Design review of the part built by this model. Coordinates are the model's own, in mm. A direction names the side the tool comes from. Give positions to 0.01 mm unless a question says otherwise; leave off trailing zeros. Loops run counter-clockwise (first coordinate to the right, second up) from the corner with the lowest first, then second, coordinate; pieces in that order, holes last. Notation, with made-up numbers: (65, 78.5) -> (75, 78.5) arc R19 cw to (75, 95.5) -> close; hole circle Ø10 at (78.25, 51.5). An arc over 180 degrees is marked (long way). Use CSV: the item, a comma, the result in double quotes. Start each with the question number.
Item 1: Clearance check with flat-ended pins moving along their axes: pin 1 (0.9 mm diameter, centred on y = -2.5, z = -4, fed in from +X) (3 decimals); pin 2 (6 mm diameter, centred on y = 17, z = -8.5, fed in from +X); pin 3 (1.4 mm diameter, centred on x = -5, y = -3.5, fed in from -Z); pin 4 (1 mm diameter, centred on y = -3.5, z = -5.5, fed in from +X). State where each tip first meets the part, or that it passes through.
Item 2: We need section C-C (y = 5.5). State the section outline as (x, z) points.
Item 3: Wall thickness on line 1 along Y through (x, z) = (2.5, -8.25); line 2 along Z through (x, y) = (10.75, 8); line 3 along Z through (x, y) = (4.5, -6): over which ranges is each line inside the solid? List them lowest first. Write a range as from..to.
Item 4: We need section A-A (y = -1). State the section outline as (x, z) points (3 decimals).
Item 5: We need section B-B (x = 0). State the section outline as (y, z) points.
Item 6: The part is to be moulded in two halves that separate along X. For faces 6 (the face through (-1.5, 15.1, 11.4)), 7 (the face through (6.875, -4, -4)), 8 (the face through (-5, -4, 3.6)), 9 (the face through (2.125, -4, -4)), say which applies: +X half, -X half, draft (parallel to the pull), parting line (faces both ways), or undercut.
Item 7: For faces 1 (the face through (11, 7, -1.1)), 2 (the face through (-9, 14.5, -5)), 3 (the face through (-5, -4, -4.4)), 4 (the face through (-6.875, -4, -4)), 5 (the face through (-4, -4, -3.6)), list the 3-axis set-ups (+Z, -Z, +X, -X, +Y, -Y) from which the entire face can be reached by the end or side of a thin tool; tool diameter is ignored.
Autodesk Inventor part; units mm, degrees
ref_plane "YZ Plane" through (0, 0, 0) normal (1, 0, 0) x (0, 1, 0)
ref_plane "XZ Plane" through (0, 0, 0) normal (0, 1, 0) x (-1, 0, 0)
ref_plane "XY Plane" through (0, 0, 0) normal (0, 0, 1) x (1, 0, 0)
sketch "Sketch1" plane through (0, 0, 0) normal (0, 1, 0) x (-1, 0, 0)
  circle A0 centre (0, 0) radius 9.9
  line L0 (-9.8387, 1.1) -> (-12.0387, 1.1)
  line L1 (-12.0387, 1.1) -> (-12.0387, -1.1)
  line L2 (-12.0387, -1.1) -> (-9.8387, -1.1)
  point P0 (-12.0387, 0)
  dimension "d0" = 19.8
  dimension "d1" = 2.2
  dimension "d2" = 2.2
extrude "Extrusion1" add sketch "Sketch1" along normal blind 14.5
sketch "Sketch2" plane through (0, 14.5, 0) normal (0, 1, 0) x (1, 0, 0)
  circle A0 centre (0, 0) radius 11.5
  dimension "d5" = 23
extrude "Extrusion2" add sketch "Sketch2" along normal blind 2
chamfer "Chamfer1" distance 0.8 angle 45 1 edges at (-11.5, 16.5, 0)
sketch "Sketch3" plane through (0, 16.5, 0) normal (0, 1, 0) x (1, 0, 0)
  circle A0 centre (0, 0) radius 10.2
  dimension "d11" = 20.4
extrude "Extrusion3" add sketch "Sketch3" along normal blind 7.5
sketch "Sketch4" plane through (0, 0, 0) normal (0, -1, 0) x (1, 0, 0)
  line L0 (-6.875, -4.4) -> (-2.125, -4.4)
  line L1 (-2.125, -4.4) -> (-2.125, -3.6)
  line L2 (-2.125, -3.6) -> (-6.875, -3.6)
  line L3 (-6.875, -3.6) -> (-6.875, -4.4)
  line L4 (2.125, -4.4) -> (6.875, -4.4)
  line L5 (6.875, -4.4) -> (6.875, -3.6)
  line L6 (6.875, -3.6) -> (2.125, -3.6)
  line L7 (2.125, -3.6) -> (2.125, -4.4)
  line L8 (-6.875, 3.6) -> (-2.125, 3.6)
  line L9 (-2.125, 3.6) -> (-2.125, 4.4)
  line L10 (-2.125, 4.4) -> (-6.875, 4.4)
  line L11 (-6.875, 4.4) -> (-6.875, 3.6)
  line L12 (-4.5, -3.6) -> (-4.5, 3.6)
  line L13 (2.125, -4) -> (-2.125, -4)
  point P0 (0, 0)
  point P1 (-4.5, -4.4)
  point P2 (4.5, -4.4)
  point P3 (-2.125, 4)
  point P4 (-4.5, 0)
  point P5 (0, -4)
  dimension "d14" = 0.8
  dimension "d15" = 4.75
  dimension "d16" = 9
  dimension "d17" = 8
extrude "Extrusion4" add sketch "Sketch4" along normal blind 9
equation "\"d2\" = d1"
properties part number "SwitchPushButton"
Results found:
1,pin 1,"x = 6.875"
1,pin 2,"x = 9.93"
1,pin 3,"z = -4.4"
1,pin 4,"through"
2,outline,"(9.84, -1.1) -> (12.04, -1.1) -> (12.04, 1.1) -> (9.84, 1.1) arc R9.9 ccw (long way) to start"
3,line 1,"0..24"
3,line 2,"-1.1..1.1"
3,line 3,"-4.4..-3.6"
4,outline,"(-6.875, -4.4) -> (-2.125, -4.4) -> (-2.125, -3.6) -> (-6.875, -3.6) -> close; (-6.875, 3.6) -> (-2.125, 3.6) -> (-2.125, 4.4) -> (-6.875, 4.4) -> close; (2.125, -4.4) -> (6.875, -4.4) -> (6.875, -3.6) -> (2.125, -3.6) -> close"
5,outline,"(0, -9.9) -> (14.5, -9.9) -> (14.5, -11.5) -> (15.7, -11.5) -> (16.5, -10.7) -> (16.5, -10.2) -> (24, -10.2) -> (24, 10.2) -> (16.5, 10.2) -> (16.5, 10.7) -> (15.7, 11.5) -> (14.5, 11.5) -> (14.5, 9.9) -> (0, 9.9) -> close"
6,face 6,"parting line"
6,face 7,"+X half"
6,face 8,"draft"
6,face 9,"undercut"
7,face 1,"-Z, +X, -Y"
7,face 2,"-Y"
7,face 3,"-Z, +X, -X, -Y"
7,face 4,"+Z, -Z, -X, -Y"
7,face 5,"+X, -X, -Y"
